Geometry: see drawing. Coordinates: mm, zero at the bounding-box minimum. A direction names the side the tool comes from. Round coordinates to 2 decimals unless told otherwise and drop trailing zeros. Loops run counter-clockwise (first coordinate to the right, second up) from the corner with the lowest first, then second, coordinate; pieces in that order, holes last. Notation, with made-up numbers: (-14, 75) - (27, 75) arc R18 ccw to (27, 80) - close; hole circle Ø8 at (86.5, 20). An arc over 180 degrees is marked (long way). Return JSON: item names as keys, results as strings. Group by question number.
1. Section D-D on y = 2.75. Return loops of the section in (x, z) (3 decimals), and give its area (3 significant figures).
2. Material intervals for probe 1 along X at (y, z) = (11, 29); probe 2 along X at (y, z) = (3.5, 27) (1 decimal); probe 3 along Y at (x, z) = (39.5, 15), sorted ascending.
3. Section C-C on z = 51. Return loops of the section in (x, y).
4. Section A-A on z = 28.75. Return loops of the section in (x, y), and give its area (3 significant figures).
5. Section B-B on x = 28.75. Return loops of the section in (y, z).
6. Set-up query: the marked faces 1 and 2. Return all of +Z, -Z, +X, -X, +Y, -Y with unobstructed straight access to the full face (end or side cutting, diameter ignored); none if empty.
7. Draft query along Z for the marked faces 3, 4 and 5. Return one class per face: +Z half, -Z half, draft (parallel to the pull), parting line (faces both ways), or undercut.
8. First-contact query: pin 1 Ø12 at (y, z) = (20.5, 35.5) entering from +X; pin 2 Ø6.5 at (x, z) = (52.5, 28.75) entering from -Y; pin 3 Ø6 at (x, y) = (24.5, 11) entering from -Z; pin 4 Ø6 at (x, y) = (18, 12) entering from -Z. Flat tips, straight axial feed; report the tip coordinate or a pass-through.
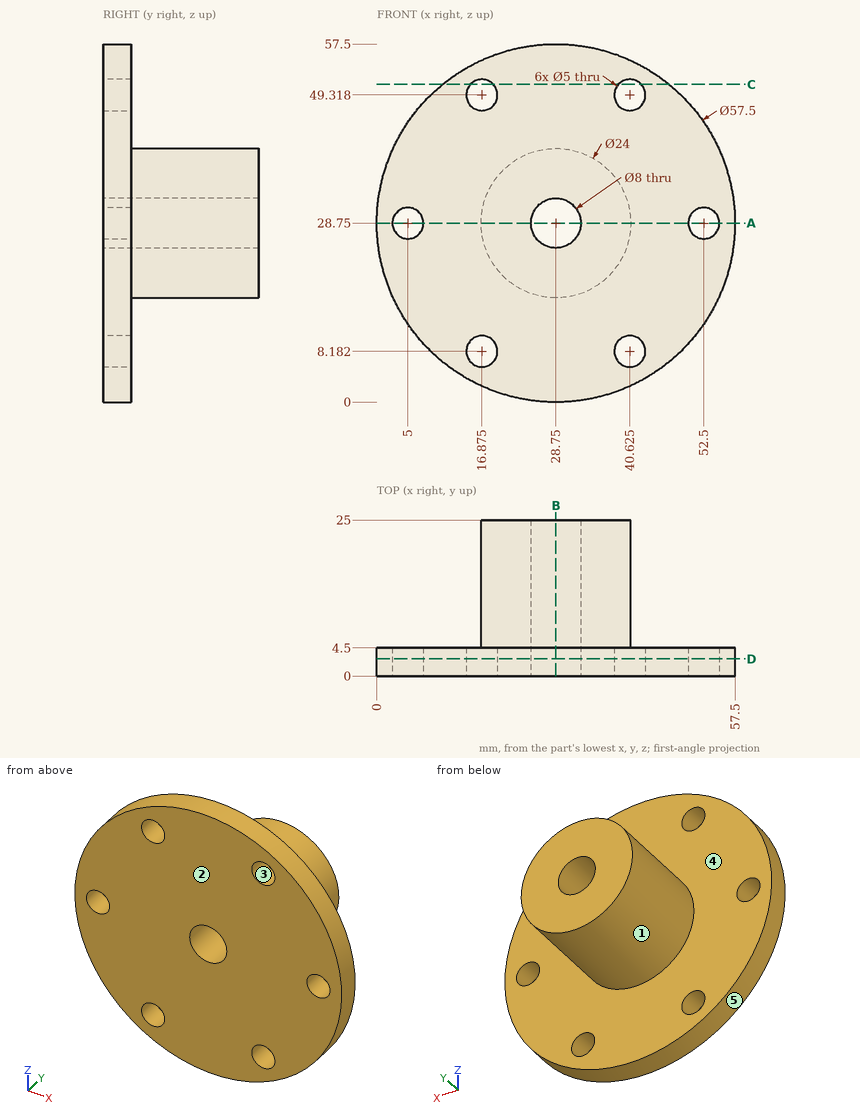
Taken from the geometry:
{
 "1": {"outline": "circle Ø57.5 at (28.75, 28.75); hole circle Ø5 at (5, 28.75); hole circle Ø5 at (16.875, 8.182); hole circle Ø5 at (16.875, 49.318); hole circle Ø8 at (28.75, 28.75); hole circle Ø5 at (40.625, 8.182); hole circle Ø5 at (40.625, 49.318); hole circle Ø5 at (52.5, 28.75)", "area": "2,430 mm2"},
 "2": {"probe 1": "16.75 to 24.76, 32.74 to 40.75", "probe 2": "0.1 to 3.2, 6.8 to 25.2, 32.3 to 50.7, 54.3 to 57.4", "probe 3": "0 to 4.5"},
 "3": {"outline": "(10.54, 0) - (15.03, 0) - (15.03, 4.5) - (10.54, 4.5) - close; (18.72, 0) - (38.78, 0) - (38.78, 4.5) - (18.72, 4.5) - close; (42.47, 0) - (46.96, 0) - (46.96, 4.5) - (42.47, 4.5) - close"},
 "4": {"outline": "(0, 0) - (2.5, 0) - (2.5, 4.5) - (0, 4.5) - close; (7.5, 0) - (24.75, 0) - (24.75, 25) - (16.75, 25) - (16.75, 4.5) - (7.5, 4.5) - close; (32.75, 0) - (50, 0) - (50, 4.5) - (40.75, 4.5) - (40.75, 25) - (32.75, 25) - close; (55, 0) - (57.5, 0) - (57.5, 4.5) - (55, 4.5) - close", "area": "506 mm2"},
 "5": {"outline": "(0, 0) - (4.5, 0) - (4.5, 16.75) - (25, 16.75) - (25, 24.75) - (0, 24.75) - close; (0, 32.75) - (25, 32.75) - (25, 40.75) - (4.5, 40.75) - (4.5, 57.5) - (0, 57.5) - close"},
 "6": {"face 1": "+Y", "face 2": "+Z, -Z, +X, -X, -Y"},
 "7": {"face 3": "undercut", "face 4": "draft", "face 5": "parting line"},
 "8": {"pin 1": "x = 40.73", "pin 2": "y = 0", "pin 3": "z = 16.82", "pin 4": "z = 19.59"}
}
